Source: three-view drawing plus pictorial views. Frame: mm from the lowest corner of the part. Coordinates: 2 decimals unless noted, no trailing zeros. Write each loop counter-clockwise with the first axis right and the second up, starting at its lowest first coordinate (ties: lowest second). Pieces come first, ordered by that corner, then holes. Notation, with made-up numbers: (-2, 53.25) - (20, 53.25) arc R15 ccw to (20, 59.25) - close; hole circle Ø4 at (-39, 35). An arc over 180 degrees is marked (long way). Answer as a JSON object with one key per item and string values. Group by question number.
Item 1: Section A-A on x = 67.5. Return loops of the section in (y, z), and give its area (3 significant figures).
Item 2: Section D-D on y = 67.5. Return loops of the section in (x, z).
Item 3: First-contact query: pin 1 Ø14.5 at (x, y) = (112.5, 67.5) entering from -Z; pin 2 Ø0.6 at (x, z) = (110.5, 1) entering from +Y; pin 3 Ø0.6 at (y, z) = (121.5, 1) entering from +X. Flat tips, straight axial feed; report the tip coordinate or a pass-through.
Item 4: Line query: line 1 along Y through (x, z) = (68, 0.95); line 2 along Y through (x, z) = (112.5, 1.3). Output: solid intervals per line, ascending. Write a range as from..to.
Item 5: Section B-B on y = 157.5. Return loops of the section in (x, z), and give its area (3 significant figures).
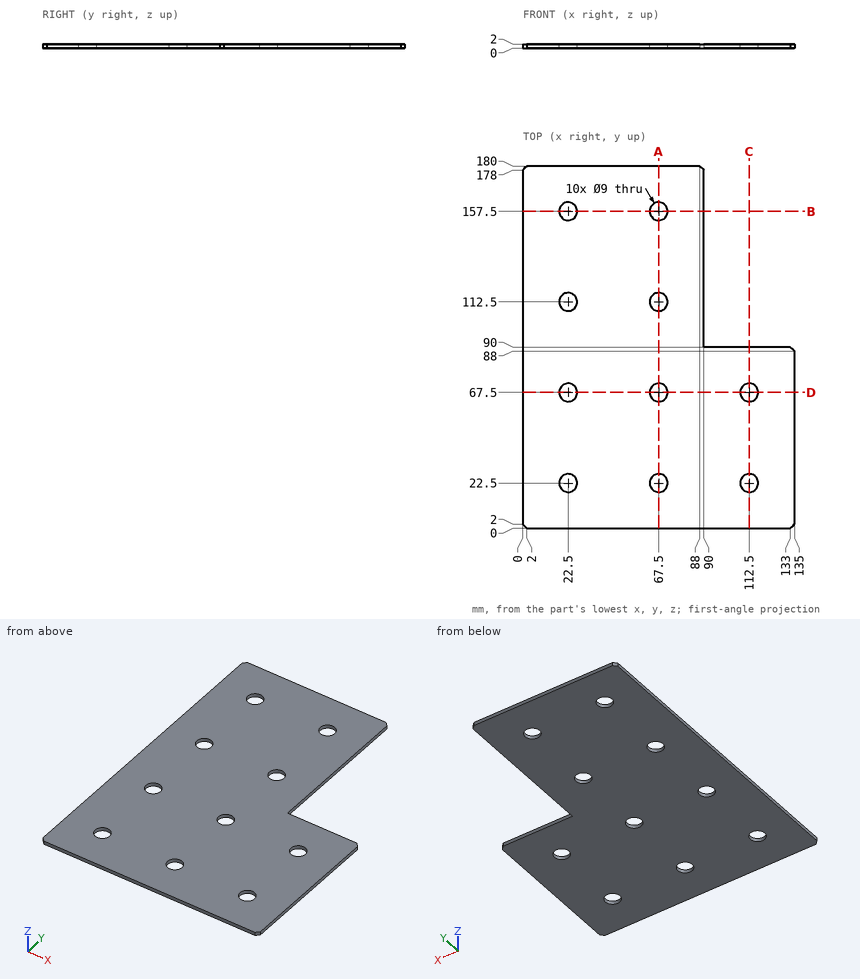
Checks:
{
 "1": {"outline": "(0, 0) - (18, 0) - (18, 2) - (0, 2) - close; (27, 0) - (63, 0) - (63, 2) - (27, 2) - close; (72, 0) - (108, 0) - (108, 2) - (72, 2) - close; (117, 0) - (153, 0) - (153, 2) - (117, 2) - close; (162, 0) - (180, 0) - (180, 2) - (162, 2) - close", "area": "288 mm^2"},
 "2": {"outline": "(0, 0) - (18, 0) - (18, 2) - (0, 2) - close; (27, 0) - (63, 0) - (63, 2) - (27, 2) - close; (72, 0) - (108, 0) - (108, 2) - (72, 2) - close; (117, 0) - (135, 0) - (135, 2) - (117, 2) - close"},
 "3": {"pin 1": "z = 0", "pin 2": "y = 90", "pin 3": "x = 90"},
 "4": {"line 1": "0..18.03, 26.97..63.03, 71.97..108.03, 116.97..153.03, 161.97..180", "line 2": "0..18, 27..63, 72..90"},
 "5": {"outline": "(0, 0) - (18, 0) - (18, 2) - (0, 2) - close; (27, 0) - (63, 0) - (63, 2) - (27, 2) - close; (72, 0) - (90, 0) - (90, 2) - (72, 2) - close", "area": "144 mm^2"}
}
